Part model, mm, in its own coordinate system. Round coordinates to 2 decimals unless told otherwise and drop trailing zeros. Loops run counter-clockwise (first coordinate to the right, second up) from the corner with the lowest first, then second, coordinate; pieces in that order, holes last.
from build123d import *

# Parameters (mm, degrees)
SKETCH_3_R      = 1.5
SKETCH_3_R_2    = 2.2
EXTRUDE_1_DEPTH = 2


with BuildPart() as part:
    # 草图3 → 凸台-拉伸1 (new body)
    with BuildSketch(Plane.XY):
        with BuildLine():
            Line((-41, -3.990216685), (-42, -3.990216685))
            Line((-42, -3.990216685), (-44, -3.990216685))
            Line((-44, -3.990216685), (-45, -3.990216685))
            Line((-45, -3.990216685), (-45, 5.009783315))
            Line((-45, 5.009783315), (-45, 15.009783315))
            Line((-45, 15.009783315), (-45, 26.463053661))
            Line((-45, 26.463053661), (-41, 30.009783315))
            ThreePointArc((-41, 30.009783315), (-34.419700864, 29.918417158), (-28.474223712, 27.097072458))
            ThreePointArc((-28.474223712, 27.097072458), (-27.224142461, 25.786703646), (-25.913822442, 24.53657125))
            ThreePointArc((-25.913822442, 24.53657125), (-15.930575492, 14.552804361), (-1.811764606, 14.552436817))
            ThreePointArc((-1.811764606, 14.552436817), (0, 14.509783437), (1.811764606, 14.552436817))
            ThreePointArc((1.811764606, 14.552436817), (15.930575492, 14.552804361), (25.913822442, 24.53657125))
            ThreePointArc((25.913822442, 24.53657125), (27.224142461, 25.786703646), (28.474223712, 27.097072458))
            ThreePointArc((28.474223712, 27.097072458), (34.419700864, 29.918417158), (41, 30.009783315))
            Line((41, 30.009783315), (45, 26.463053661))
            Line((45, 26.463053661), (45, 15.009783315))
            Line((45, 15.009783315), (45, 5.009783315))
            Line((45, 5.009783315), (45, -2.990216685))
            ThreePointArc((45, -2.990216685), (44, -2.990216685), (44, -3.990216685))
            Line((44, -3.990216685), (41, -3.990216685))
            Line((41, -3.990216685), (27.7, -3.990216685))
            ThreePointArc((27.7, -3.990216685), (26.285786438, -3.404430248), (25.7, -1.990216685))
            Line((25.7, -1.990216685), (25.7, 5.024732502))
            ThreePointArc((25.7, 5.024732502), (25.114213562, 6.438946065), (23.7, 7.024732502))
            Line((23.7, 7.024732502), (-23.7, 7.024732502))
            ThreePointArc((-23.7, 7.024732502), (-25.114213562, 6.438946065), (-25.7, 5.024732502))
            Line((-25.7, 5.024732502), (-25.7, -1.990216685))
            ThreePointArc((-25.7, -1.990216685), (-26.285786438, -3.404430248), (-27.7, -3.990216685))
            Line((-27.7, -3.990216685), (-41, -3.990216685))
        make_face()
        with Locations((42, 10.009783315)):
            Circle(SKETCH_3_R, mode=Mode.SUBTRACT)
        with Locations(Location((-42, 10.009783315, 0), (0, 0, 180))):
            Circle(SKETCH_3_R, mode=Mode.SUBTRACT)
        with Locations((0, 11.009783312)):
            Circle(SKETCH_3_R_2, mode=Mode.SUBTRACT)
        with Locations((-29.69848481, 23.311298502)):
            Circle(SKETCH_3_R_2, mode=Mode.SUBTRACT)
        with Locations((29.69848481, 23.311298502)):
            Circle(SKETCH_3_R_2, mode=Mode.SUBTRACT)
        with BuildLine():
            Line((-37.1, -2.090216685), (-29.9, -2.090216685))
            Line((-29.9, -2.090216685), (-29.9, 0.109783315))
            Line((-29.9, 0.109783315), (-37.1, 0.109783315))
            ThreePointArc((-37.1, 0.109783315), (-37.555634919, -0.990216685), (-37.1, -2.090216685))
        make_face(mode=Mode.SUBTRACT)
        with BuildLine():
            Line((29.9, -2.090216685), (29.9, 0.109783315))
            Line((29.9, 0.109783315), (37.1, 0.109783315))
            ThreePointArc((37.1, 0.109783315), (37.555634919, -0.990216685), (37.1, -2.090216685))
            Line((37.1, -2.090216685), (29.9, -2.090216685))
        make_face(mode=Mode.SUBTRACT)
        with BuildLine():
            Line((-43.1, 5.109783315), (-43.1, -0.090216685))
            Line((-43.1, -0.090216685), (-40.9, -0.090216685))
            Line((-40.9, -0.090216685), (-40.9, 5.109783315))
            ThreePointArc((-40.9, 5.109783315), (-42, 5.565418233), (-43.1, 5.109783315))
        make_face(mode=Mode.SUBTRACT)
        with BuildLine():
            Line((-43.1, 20.109783315), (-40.9, 20.109783315))
            Line((-40.9, 20.109783315), (-40.9, 14.909783315))
            ThreePointArc((-40.9, 14.909783315), (-42, 14.454148396), (-43.1, 14.909783315))
            Line((-43.1, 14.909783315), (-43.1, 20.109783315))
        make_face(mode=Mode.SUBTRACT)
        with BuildLine():
            Line((40.9, 20.109783315), (40.9, 14.909783315))
            ThreePointArc((40.9, 14.909783315), (42, 14.454148396), (43.1, 14.909783315))
            Line((43.1, 14.909783315), (43.1, 20.109783315))
            Line((43.1, 20.109783315), (40.9, 20.109783315))
        make_face(mode=Mode.SUBTRACT)
        with BuildLine():
            Line((40.9, 5.109783315), (40.9, -0.090216685))
            Line((40.9, -0.090216685), (43.1, -0.090216685))
            Line((43.1, -0.090216685), (43.1, 5.109783315))
            ThreePointArc((43.1, 5.109783315), (42, 5.565418233), (40.9, 5.109783315))
        make_face(mode=Mode.SUBTRACT)
    extrude(amount=EXTRUDE_1_DEPTH)


solid = part.part
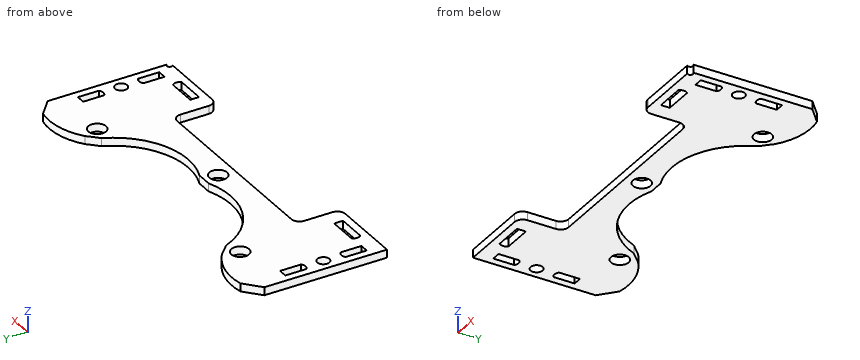
1) Wall check: line 1 along X through (y, z) = (3.5, 1.05); line 2 along X through (y, z) = (-1, 1.05); line 3 along Y through (x, z) = (41, 0.6). Give the ranges that are in metal, low to high.
Values:
line 1: x = -45 to -43.1, -40.9 to -25.7, 25.7 to 40.9, 43.1 to 45
line 2: x = -45 to -37.56, -29.9 to -25.7, 25.7 to 29.9, 37.56 to 45
line 3: y = -3.99 to -0.09, 5.2 to 8.89, 11.13 to 14.82, 20.11 to 30.01
2) Slice it at B-B, the plane x = 42. Give the cut face in (y, z).
Values:
outline: (-3.99, 0) - (-0.09, 0) - (-0.09, 2) - (-3.99, 2) - close; (5.57, 0) - (8.51, 0) - (8.51, 2) - (5.57, 2) - close; (11.51, 0) - (14.45, 0) - (14.45, 2) - (11.51, 2) - close; (20.11, 0) - (29.12, 0) - (29.12, 2) - (20.11, 2) - close
3) Slice it at A-A, the plane x = 0. Give the cut face in (y, z), then the cut area to 3 significant figures.
Values:
outline: (7.02, 0) - (8.81, 0) - (8.81, 2) - (7.02, 2) - close; (13.21, 0) - (14.51, 0) - (14.51, 2) - (13.21, 2) - close
area: 6.17 mm2
4) Drop flat-ended pins along their axis: pin 1 Ø3.5 at (x, y) = (42, 10.01) entering from +Z; pin 2 Ø4 at (x, y) = (0, 11.01) entering from -Z; pin 3 Ø0.6 at (x, z) = (34.5, 0.5) entering from +Y. Give the stop position or say it passes through.
Values:
pin 1: stops at z = 2
pin 2: passes through
pin 3: stops at y = 30
5) Slice it at C-C, the plane z = 0.4. Give the number of separate pieces and of enclosed holes in the cut face, then the cut area to 3 significant figures.
Values:
separate pieces: 1
enclosed holes: 11
area: 1,550 mm2
6) Slice it at D-D, the plane x = 9.5. Give the cut face in (y, z), then the cut area to 3 significant figures.
Values:
outline: (7.02, 0) - (13.16, 0) - (13.16, 2) - (7.02, 2) - close
area: 12.3 mm2
